Geometry: final body of the model. Coordinates: model frame, mm. Face numbers are marked on the shaded views. A direction names the side the tool comes from. Give positions to 0.01 mm unless a question says otherwise; leave off trailing zeros. Write each loop counter-clockwise with the first axis right and the second up, starting at its lowest first coordinate (ties: lowest second). Pieces come first, ordered by that corner, then holes. Notation, with made-up numbers: (32, -19) -> (83, -19) arc R5 ccw to (83, -11) -> close; hole circle Ø3 at (85.25, 89). An arc over 180 degrees is marked (long way). Answer in a Markdown table with one row per item. Add a question column.
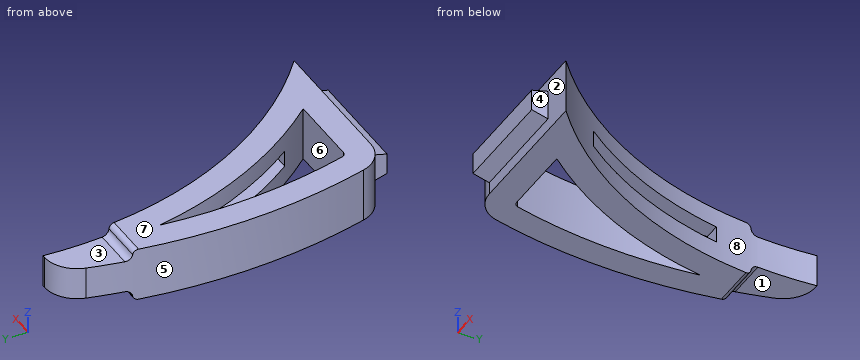
from build123d import *

# Parameters (mm, degrees)
BOSS_EXTRU_1_DEPTH      = 10
ENL_V_START             = 3
ESQUISSE3_W             = 3
ESQUISSE3_H             = 30
ENL_V_MAT_EXTRU_2_DEPTH = 66.07803068
BOSS_EXTRU_2_START      = 4.5
BOSS_EXTRU_2_DEPTH      = 20
ENL_V_MAT_EXTRU_3_DEPTH = 2
ENL_V_MAT_EXTRU_3_TAPER = -30
CONG_1_R                = 1.325
CONG_2_R                = 1.325
CONG_VARIABLE1_R        = 1


with BuildPart() as part:
    # Esquisse1 → Boss.-Extru.1 (new body)
    with BuildSketch(Plane.XY):
        with BuildLine():
            Line((4.509378002, 0), (30.57152697, 0))
            ThreePointArc((30.57152697, 0), (10.370789772, 26.839796662), (5, 60))
            Line((5, 60), (4.509378002, 60))
            ThreePointArc((4.509378002, 60), (0.848195772, 58.753498152), (-1.291762986, 55.531914894))
            ThreePointArc((-1.291762986, 55.531914894), (-4.606079858, 30), (-1.291762986, 4.468085106))
            ThreePointArc((-1.291762986, 4.468085106), (0.848195772, 1.246501848), (4.509378002, 0))
        make_face()
        with BuildLine():
            Line((4.509378002, 5), (18.232904672, 5))
            ThreePointArc((18.232904672, 5), (7.212441996, 21.704317491), (1.001630768, 40.728266722))
            ThreePointArc((1.001630768, 40.728266722), (0.643507572, 23.118189348), (3.54252117, 5.744680851))
            ThreePointArc((3.54252117, 5.744680851), (3.899180963, 5.207750308), (4.509378002, 5))
        make_face(mode=Mode.SUBTRACT)
    extrude(amount=BOSS_EXTRU_1_DEPTH)

    # Esquisse3 → Enlèv. mat.-Extru.2 (cut, through all)
    with BuildSketch(Plane(origin=(0, 0, 0), x_dir=(0, 0, -1), z_dir=(1, 0, 0)).offset(ENL_V_START)):
        with Locations((-5, 25.901656599)):
            Rectangle(ESQUISSE3_W, ESQUISSE3_H)
    extrude(amount=ENL_V_MAT_EXTRU_2_DEPTH, mode=Mode.SUBTRACT)


with BuildPart() as boss_extru_2_tool:
    # Esquisse4 → Boss.-Extru.2 (new body)
    with BuildSketch(Plane(origin=(0, 0, 0), x_dir=(0, 0, -1), z_dir=(1, 0, 0)).offset(BOSS_EXTRU_2_START)):
        Polygon((-7.75, 0), (-2.25, 0), (-3.053847577, -3), (-6.946152423, -3), align=None)
    extrude(amount=BOSS_EXTRU_2_DEPTH)


with BuildPart() as part_1:
    add(part.part)


with BuildPart() as part_2:
    # Boss.-Extru.2: joined with boss_extru_2_tool
    add(part_1.part.fuse(boss_extru_2_tool.part, tol=0.00001))

    # Esquisse6 → Enlèv. mat.-Extru.3 (cut)
    with BuildSketch(Plane.XY):
        with BuildLine():
            Line((-2.972740877, 48), (5.048977769, 48))
            ThreePointArc((5.048977769, 48), (4.766869828, 53.998948533), (5, 60))
            Line((5, 60), (4.509378002, 60))
            ThreePointArc((4.509378002, 60), (0.848195772, 58.753498152), (-1.291762986, 55.531914894))
            ThreePointArc((-1.291762986, 55.531914894), (-2.204935767, 51.782179075), (-2.972740877, 48))
        make_face()
    enl_v_mat_extru_3 = extrude(amount=ENL_V_MAT_EXTRU_3_DEPTH, taper=ENL_V_MAT_EXTRU_3_TAPER, mode=Mode.SUBTRACT)

    # Symétrie1: Enlèv. mat.-Extru.3 across plane
    add(enl_v_mat_extru_3.mirror(Plane(origin=(0, 0, 5), x_dir=(1, 0, 0), z_dir=(0, 0, -1))), mode=Mode.SUBTRACT)

    # Congé1
    cong_1_edges = [part_2.edges().sort_by_distance(p)[0] for p in [
        (0.992837273, 46.845299462, 8),
    ]]
    fillet(cong_1_edges, radius=CONG_1_R)

    # Congé2
    cong_2_edges = [part_2.edges().sort_by_distance(p)[0] for p in [
        (0.992837273, 46.845299462, 2),
    ]]
    fillet(cong_2_edges, radius=CONG_2_R)

    # Congé variable1
    cong_variable1_edges = [part_2.edges().sort_by_distance(p)[0] for p in [
        (1.038118446, 48, 0),
        (1.038118446, 48, 10),
    ]]
    fillet(cong_variable1_edges, radius=CONG_VARIABLE1_R)


solid = part_2.part
Q1. Pull-direction query (X, two-part tool) for the marked faces 6, 7 and 8; classes: +X half, -X half, draft (parallel to the pull), parting line (faces both ways), or undercut.
Q2. Contact query for flat-ended pins moving along their axis: pin 1 Ø4 at (x, y) = (1, 57) entering from +Z; pin 2 Ø5 at (x, y) = (10.5, 28.5) entering from +Z; pin 3 Ø2 at (y, z) = (37.5, 9) entering from +X; pin 4 Ø6 at (x, y) = (-0.5, 56.5) entering from -Z. Output: stop coordinate, or through.
Q3. Section C-C on y = 8. Return loops of the section in (x, z).
Q4. Section A-A on x = 10. Return loops of the section in (y, z).
Q5. Line query: probe 1 along Z at (x, y) = (8.5, 25.5); probe 2 along X at (y, z) = (15, 2.25); probe 3 along X at (y, z) = (27, 9.25). Output: solid intervals per line, ascending. Write a range as from..to.
Q6. Section B-B on y = 28.5. Return loops of the section in (x, z).
Q7. Access query for the marked faces 1, 2, 3, 4 and 5. Directions: +Z, -Z, +X, -X, +Y, -Y. A direction counts if a zero-diameter tool reaches every point of the face in a straight line with its end or side. Return the directions, or none.
Q8. Section D-D on x = 21. Return loops of the section in (y, z), and give its area (3 significant figures).
Checks:
| question | item | result |
|---|---|---|
| 1 | face 6 | undercut |
| 1 | face 7 | draft |
| 1 | face 8 | +X half |
| 2 | pin 1 | z = 8 |
| 2 | pin 2 | z = 10 |
| 2 | pin 3 | x = 7.06 |
| 2 | pin 4 | z = 2 |
| 3 | outline | (-2.16, 0) -> (2.98, 0) -> (2.98, 10) -> (-2.16, 10) -> close; (15.75, 0) -> (22.25, 0) -> (22.25, 10) -> (15.75, 10) -> close |
| 4 | outline | (-3, 3.05) -> (0, 2.25) -> (0, 0) -> (5, 0) -> (5, 10) -> (0, 10) -> (0, 7.75) -> (-3, 6.95) -> close; (16.46, 0) -> (27.73, 0) -> (27.73, 3.5) -> (16.46, 3.5) -> close; (16.46, 6.5) -> (27.73, 6.5) -> (27.73, 10) -> (16.46, 10) -> close |
| 5 | probe 1 | 0..3.5, 6.5..10 |
| 5 | probe 2 | -3.47..1.59, 10.88..16.83 |
| 5 | probe 3 | -4.56..0.44, 4.91..10.3 |
| 6 | outline | (-4.59, 0) -> (0.41, 0) -> (0.41, 10) -> (-4.59, 10) -> close; (4.34, 0) -> (9.69, 0) -> (9.69, 3.5) -> (4.34, 3.5) -> close; (4.34, 6.5) -> (9.69, 6.5) -> (9.69, 10) -> (4.34, 10) -> close |
| 7 | face 1 | -Z, +X, -X, +Y |
| 7 | face 2 | +X, -Y |
| 7 | face 3 | +Z, +X, -X, +Y |
| 7 | face 4 | +Z, -Z, +X, -Y |
| 7 | face 5 | +Z, -Z, -X |
| 8 | outline | (-3, 3.05) -> (0, 2.25) -> (0, 0) -> (9.46, 0) -> (9.46, 10) -> (0, 10) -> (0, 7.75) -> (-3, 6.95) -> close |
| 8 | area | 109 mm^2 |
